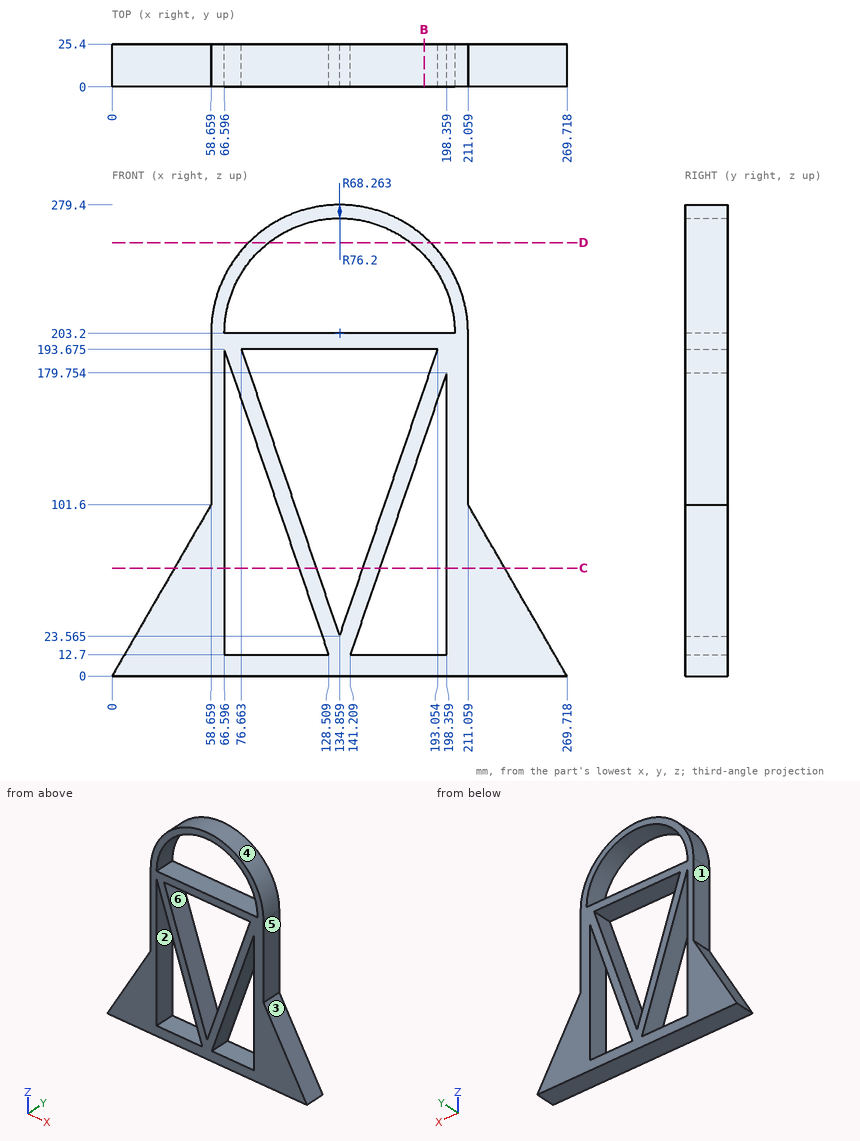
Design review of the part shown in the three views and the two pictorial views. Dimensions are in mm from the part's minimum x, y and z. A direction names the side the tool comes from. Round coordinates to 2 decimals unless told otherwise and drop trailing zeros. Loops run counter-clockwise (first coordinate to the right, second up) from the corner with the lowest first, then second, coordinate; pieces in that order, holes last.
1) Consider section D-D on z = 257. State the section outline as (x, y) points (1 decimal), then the cut area to 3 significant figures.
Values follow:
outline: (80.9, 0) - (92.8, 0) - (92.8, 25.4) - (80.9, 25.4) - close; (176.9, 0) - (188.8, 0) - (188.8, 25.4) - (176.9, 25.4) - close
area: 607 mm2
2) Consider section B-B on x = 185. State the section outline as (y, z) points (1 decimal).
Values follow:
outline: (0, 0) - (25.4, 0) - (25.4, 12.7) - (0, 12.7) - close; (0, 140.7) - (25.4, 140.7) - (25.4, 170.1) - (0, 170.1) - close; (0, 193.7) - (25.4, 193.7) - (25.4, 203.2) - (0, 203.2) - close; (0, 249.5) - (25.4, 249.5) - (25.4, 260.6) - (0, 260.6) - close
3) Wall thickness on line 1 along X through (y, z) = (21.5, 67.5) (1 decimal); line 2 along X through (y, z) = (17.5, 71) (1 decimal); line 3 along X through (y, z) = (23.75, 264.5) (1 decimal): over which ranges is each line inside the solid? List them lowest first.
Values follow:
line 1: x = 39 to 66.6, 109.8 to 119.8, 149.9 to 160, 198.4 to 230.7
line 2: x = 41 to 66.6, 108.6 to 118.6, 151.1 to 161.2, 198.4 to 228.7
line 3: x = 89.6 to 104.8, 164.9 to 180.1
4) Tool access review of the marked faces 1, 2 and 3: name each direction out of +Z, -Z, +X, -X, +Y, -Y from which nothing blocks a thin tool from reaching the whole face with its end or side.
Values follow:
face 1: +Z, -X, +Y, -Y
face 2: +Y, -Y
face 3: +Z, +X, +Y, -Y
5) Consider section C-C on z = 64. Give the number of separate pieces and of enclosed holes in the cut face, then the cut area to 3 significant figures.
Values follow:
separate pieces: 4
enclosed holes: 0
area: 2,140 mm2
6) Clearance check with flat-ended pins moving along their axes: P1, Ø12.5, axis at y = 6.5, z = 143, coming from the +X side; P2, Ø1.5, axis at y = 9, z = 182.5, coming from the -X side; P3, Ø7.5, axis at x = 113.5, y = 11, coming from the +Z side. State where each tip first meets the part, or that it passes through.
Values follow:
P1: stops at x = 211.06
P2: stops at x = 58.66
P3: stops at z = 277.34
7) The part is to be moulded in two halves that separate along X. For the marked faces 4, 5 and 6, say which applies: pulls with the +X half, pulls with the -X half, needs draft (parallel to the pull), parting line crosses it, or undercut.
Values follow:
face 4: parting line crosses it
face 5: pulls with the +X half
face 6: undercut
